For this review, use the dimensioned drawing (mm, ordinates from the lowest corner) and the shaded views. Coordinates: 2 decimals unless noted, no trailing zeros. Loops run counter-clockwise (first coordinate to the right, second up) from the corner with the lowest first, then second, coordinate; pieces in that order, holes last. Notation, with made-up numbers: (64, 9.25) -> (98, 9.25) arc R33 ccw to (98, 37.25) -> close; hole circle Ø2 at (22.5, 36.5). An arc over 180 degrees is marked (long way). Use one line per item in the form item = value. Start each with the question number.
1. Wall thickness on line 1 (Y direction, x = 49, z = 1.2) (3 decimals); line 2 (Z direction, x = 3.5, y = 2); line 3 (Y direction, x = 34.5, z = 16.25): over which ranges is each line inside the solid? List them lowest first. Write a range as from..to.
2. Consider section C-C (z = 9.75). State the section outline as (x, y) points, then the cut area to 3 significant figures.
3. Consider section D-D (y = 0.5). State the section outline as (x, z) points, then the cut area to 3 significant figures.
4. For pin 1 (2.5 mm diameter, centred on x = 45, y = 4, fed in from +Z); pin 2 (0.8 mm diameter, centred on y = 0.5, z = 9.5, fed in from +X); pin 3 (4 mm diameter, centred on y = 1.5, z = 15, fed in from +X), all flat-tipped, find the tip position at first contact; note any pin that passes through.
5. The part is to be moulded in two halves that separate along X. For the marked faces 1 and 2, say which applies: released by +X, released by -X, zero draft, split by the parting line, or undercut.
6. Consider section B-B (y = 6). State how many separate pieces and enclosed holes the cut face has.
7. Consider section A-A (x = 49). State the section outline as (y, z) points (3 decimals), then the cut area to 3 significant figures.
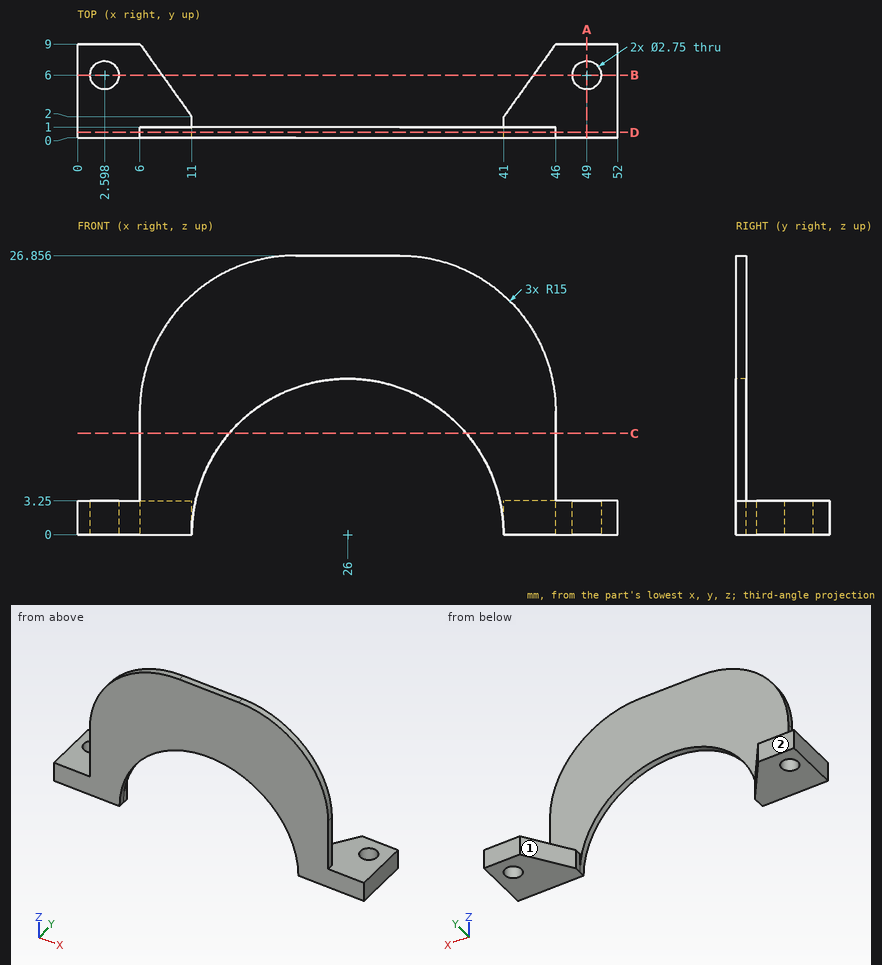
Geometry check:
q1.line_1 = 0..4.625, 7.375..9
q1.line_2 = 0..3.25
q1.line_3 = 0..1
q2.outline = (6, 0) -> (14.6, 0) -> (14.6, 1) -> (6, 1) -> close; (37.4, 0) -> (46, 0) -> (46, 1) -> (37.4, 1) -> close
q2.area = 17.2 mm²
q3.outline = (0, 0) -> (11, 0) arc R15 cw to (41, 0) -> (52, 0) -> (52, 3.25) -> (46, 3.25) -> (46, 11.86) arc R15 ccw to (31, 26.86) -> (21, 26.86) arc R15 ccw to (6, 11.86) -> (6, 3.25) -> (0, 3.25) -> close
q3.area = 663 mm²
q4.pin_1 = 3.25
q4.pin_2 = 46
q4.pin_3 = 45.95
q5.face_1 = undercut
q5.face_2 = zero draft
q6.separate_pieces = 4
q6.enclosed_holes = 0
q7.outline = (0, 0) -> (4.625, 0) -> (4.625, 3.25) -> (0, 3.25) -> close; (7.375, 0) -> (9, 0) -> (9, 3.25) -> (7.375, 3.25) -> close
q7.area = 20.3 mm²
